```python
from build123d import *

# Parameters (mm, degrees)
SKETCH1_W           = 230
SKETCH1_H           = 300
SKETCH1_R           = 5.5
BOSS_EXTRUDE1_DEPTH = 6


with BuildPart() as part:
    # Sketch1 → Boss-Extrude1 (new body)
    with BuildSketch(Plane(origin=(0, 0, 0), x_dir=(1, 0, 0), z_dir=(0, 1, 0))):
        with Locations((115, 150)):
            Rectangle(SKETCH1_W, SKETCH1_H)
        with Locations(Location((15, 15, 0), (0, 0, 270))):
            Circle(SKETCH1_R, mode=Mode.SUBTRACT)
        with Locations(Location((15, 285, 0), (0, 0, 270))):
            Circle(SKETCH1_R, mode=Mode.SUBTRACT)
        with Locations(Location((15, 150, 0), (0, 0, 270))):
            Circle(SKETCH1_R, mode=Mode.SUBTRACT)
        with Locations(Location((215, 15, 0), (0, 0, 90))):
            Circle(SKETCH1_R, mode=Mode.SUBTRACT)
        with Locations(Location((215, 150, 0), (0, 0, 90))):
            Circle(SKETCH1_R, mode=Mode.SUBTRACT)
        with Locations(Location((215, 285, 0), (0, 0, 90))):
            Circle(SKETCH1_R, mode=Mode.SUBTRACT)
        with Locations(Location((165, 15, 0), (0, 0, 90))):
            Circle(SKETCH1_R, mode=Mode.SUBTRACT)
        with Locations(Location((115, 15, 0), (0, 0, 90))):
            Circle(SKETCH1_R, mode=Mode.SUBTRACT)
        with Locations(Location((65, 15, 0), (0, 0, 90))):
            Circle(SKETCH1_R, mode=Mode.SUBTRACT)
        with Locations(Location((165, 285, 0), (0, 0, 90))):
            Circle(SKETCH1_R, mode=Mode.SUBTRACT)
        with Locations(Location((115, 285, 0), (0, 0, 90))):
            Circle(SKETCH1_R, mode=Mode.SUBTRACT)
        with Locations(Location((65, 285, 0), (0, 0, 90))):
            Circle(SKETCH1_R, mode=Mode.SUBTRACT)
    extrude(amount=BOSS_EXTRUDE1_DEPTH)


solid = part.part
```
Design review of the part built by this model. Coordinates are the model's own, in mm. Coordinates: 2 decimals unless noted, no trailing zeros. Loops run counter-clockwise (first coordinate to the right, second up) from the corner with the lowest first, then second, coordinate; pieces in that order, holes last. Notation, with made-up numbers: M -21.5,49.25 L -11.5,49.25 A23 ccw -11.5,67.25 Z; hole C -3.75,71 d2. An arc over 180 degrees is marked long. One line per question, with ' | ' between items.
(1) We need section A-A (x = 215). Give the boundary of the cut face in (y, z).
Filled in:
outline: M 0,-300 L 6,-300 L 6,-290.5 L 0,-290.5 Z; M 0,-279.5 L 6,-279.5 L 6,-155.5 L 0,-155.5 Z; M 0,-144.5 L 6,-144.5 L 6,-20.5 L 0,-20.5 Z; M 0,-9.5 L 6,-9.5 L 6,0 L 0,0 Z
(2) Draft analysis for pull direction Z (two halves, no side actions). For faces 1 (the face through (113, 3, 0)), 2 (the face through (220.37, 2.96, -13.81)), 3 (the face through (113, 0, -152)), state which applies: released by +Z, released by -Z, zero draft, split by the parting line, or undercut.
Filled in:
face 1: released by +Z | face 2: undercut | face 3: zero draft
(3) Wall thickness on probe 1 along X at (y, z) = (2.1, -285); probe 2 along Z at (x, y) = (165, 1.25): over which ranges is each line inside the solid? List them lowest first.
Filled in:
probe 1: x = 0 to 9.5, 20.5 to 59.5, 70.5 to 109.5, 120.5 to 159.5, 170.5 to 209.5, 220.5 to 230 | probe 2: z = -300 to -290.5, -279.5 to -20.5, -9.5 to 0
(4) We need section C-C (z = -15). Give the boundary of the cut face in (x, y).
Filled in:
outline: M 0,0 L 9.5,0 L 9.5,6 L 0,6 Z; M 20.5,0 L 59.5,0 L 59.5,6 L 20.5,6 Z; M 70.5,0 L 109.5,0 L 109.5,6 L 70.5,6 Z; M 120.5,0 L 159.5,0 L 159.5,6 L 120.5,6 Z; M 170.5,0 L 209.5,0 L 209.5,6 L 170.5,6 Z; M 220.5,0 L 230,0 L 230,6 L 220.5,6 Z
(5) For pin 1 Ø10 at (x, z) = (15, -15) entering from +Y, flat-tipped, find the tip position at first contact; note if it passes through.
Filled in:
pin 1: passes through
(6) We need section B-B (y = 2.8). Count the separate pieces of the cut face and the enclosed holes in it, and give its area (3 significant figures).
Filled in:
separate pieces: 1 | enclosed holes: 12 | area: 67,900 mm^2
(7) We need section D-D (x = 165). Give the boundary of the cut face in (y, z).
Filled in:
outline: M 0,-300 L 6,-300 L 6,-290.5 L 0,-290.5 Z; M 0,-279.5 L 6,-279.5 L 6,-20.5 L 0,-20.5 Z; M 0,-9.5 L 6,-9.5 L 6,0 L 0,0 Z
